Part model, mm, in its own coordinate system. Give positions to 0.01 mm unless a question says otherwise; leave off trailing zeros. Order: outer loops, then holes, each group sorted by start corner. A loop starts at its lowest first (then second) coordinate and runs counter-clockwise, first axis right, second up.
1. Slice it at C-C on x = 42. List the corners of the cut face in (y, z), and give its area (3 significant figures).
2. Drop flat-ended pins along their axis: pin 1 Ø1.5 at (y, z) = (-23.5, 11.5) entering from +X; pin 2 Ø1.5 at (y, z) = (-13, 18) entering from +X; pin 3 Ø1 at (x, z) = (29, 21.5) entering from +Y. Give the stop position or say it passes through.
3. Slice it at B-B on y = -12.5. List the corners of the cut face in (x, z).
4. Slice it at A-A on z = 12.25. List the corners of the cut face in (x, y).
5. Probe line 1 (X direction, y = -1, z = 1.5); line 2 (X direction, y = -24, z = 11.75); line 3 (Y direction, x = 41, z = 21.25). List the from-to ranges inside material, lowest first.
from build123d import *

# Parameters (mm, degrees)
F1_DEPTH = 25.4
F2_SIZE  = 8.89


with BuildPart() as f1:
    # F0 (on Top) → F1 (new body)
    with BuildSketch(Plane.XY):
        Polygon((44.037506, 0), (0, 0), (0, -27.267408), (49.926244, -27.267408), align=None)
    extrude(amount=F1_DEPTH)

    # F2
    f2_edges = [f1.edges().sort_by_distance(p)[0] for p in [
        (44.037506, 0, 12.7),
    ]]
    chamfer(f2_edges, length=F2_SIZE)


solid = f1.part
Data:
1. outline: (-27.27, 0) - (-5.53, 0) - (-5.53, 25.4) - (-27.27, 25.4) - close
1. area: 552 mm2
2. pin 1: stops at x = 49.27
2. pin 2: stops at x = 47.01
2. pin 3: stops at y = 0
3. outline: (0, 0) - (46.74, 0) - (46.74, 25.4) - (0, 25.4) - close
4. outline: (0, -27.27) - (49.93, -27.27) - (45.91, -8.69) - (35.15, 0) - (0, 0) - close
5. line 1: x = 0 to 36.39
5. line 2: x = 0 to 49.22
5. line 3: y = -27.27 to -4.72
